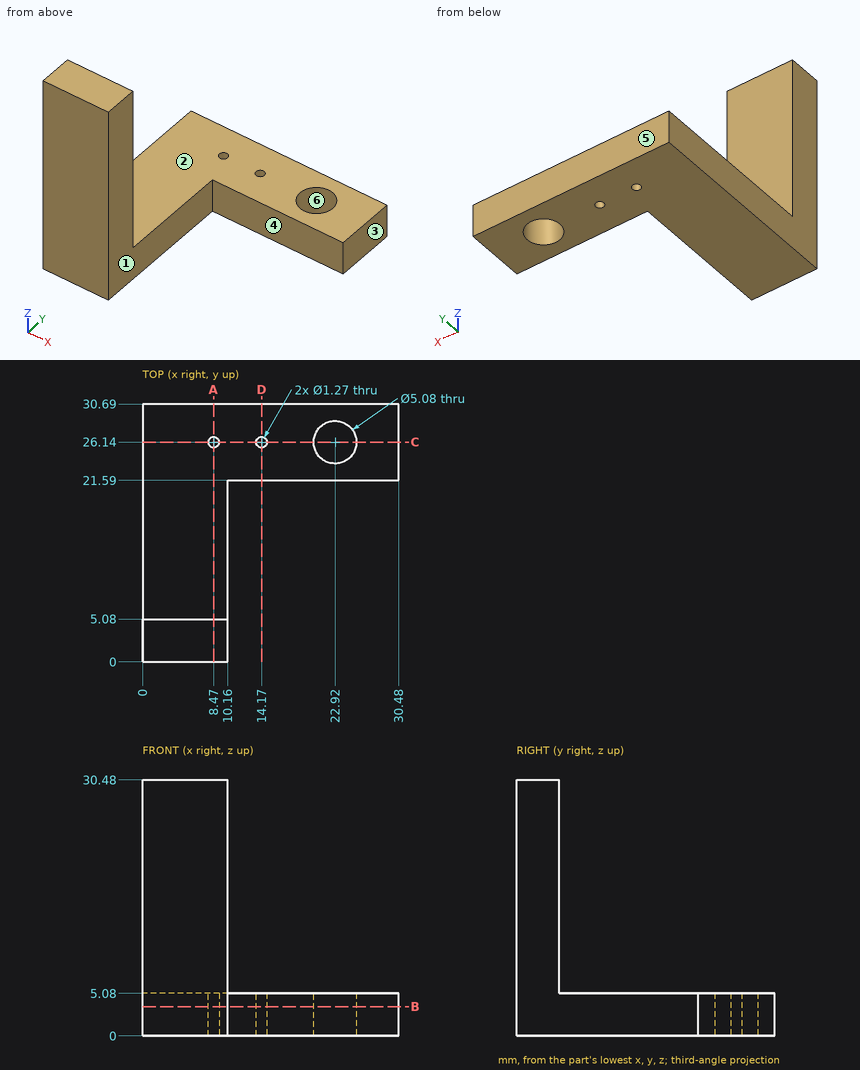
Print and shaded views of the part. All mm, measured from the part's lowest x, y and z. A direction names the side the tool comes from. Give positions to 0.01 mm unless a question says otherwise; leave off trailing zeros. Loops run counter-clockwise (first coordinate to the right, second up) from the corner with the lowest first, then second, coordinate; pieces in that order, holes last. Notation, with made-up numbers: (50.5, 1.5) - (67.5, 1.5) arc R29 cw to (67.5, 38.5) - close; hole circle Ø2 at (-15, -6.75). An arc over 180 degrees is marked (long way). One line per item, written item: value. Start each with the question number.
1. Slice it at D-D (x = 14.17). List the corners of the cut face in (y, z) (3 decimals).
2. Pin check, flat tips, straight feed: pin 1 (3 mm diameter, centred on x = 13, z = 7, fed in from -Y); pin 2 (2 mm diameter, centred on x = 8.47, y = 26.14, fed in from +Z); pin 3 (4 mm diameter, centred on x = 23, z = 3, fed in from -Y); pin 4 (5 mm diameter, centred on x = 3, z = 12, fed in from +Y). Stop position of each tip, or through.
3. Slice it at B-B (z = 3.5). List the corners of the cut face in (x, y) (3 decimals).
4. Probe L1, parallel to Y at x = 22.92, z = 3.4; L2, parallel to Y at x = 8.47, z = 1.8 (3 decimals); L3, parallel to X at y = 26, z = 2. List the from-to ranges inside material, lowest first. Write a range as from..to.
5. Slice it at A-A (x = 8.47). List the corners of the cut face in (y, z) (3 decimals), plus the area to 3 significant figures.
6. Pull direction Y, two halves, no side cores. Call the marked faces 4, 5 and 6: pulls with the +Y half, pulls with the -Y half, needs draft (parallel to the pull), parting line crosses it, or undercut.
7. Which spindle directions (+Z, -Z, +X, -X, +Y, -Y) get a long thin tool onto all of the face, cutting with end or side? Do the marked faces 1, 2 and 3. Say none if no direction does.
8. Slice it at C-C (y = 26.14). List the corners of the cut face in (x, z) (3 decimals), plus the area to 3 significant figures.
Solution:
1. outline: (21.59, 0) - (25.505, 0) - (25.505, 5.08) - (21.59, 5.08) - close; (26.775, 0) - (30.69, 0) - (30.69, 5.08) - (26.775, 5.08) - close
2. pin 1: passes through
2. pin 2: stops at z = 5.08
2. pin 3: stops at y = 21.59
2. pin 4: stops at y = 5.08
3. outline: (0, 0) - (10.16, 0) - (10.16, 21.59) - (30.48, 21.59) - (30.48, 30.69) - (0, 30.69) - close; hole circle Ø1.27 at (8.47, 26.14); hole circle Ø1.27 at (14.17, 26.14); hole circle Ø5.08 at (22.92, 26.14)
4. L1: y = 21.59..23.6, 28.68..30.69
4. L2: y = 0..25.505, 26.775..30.69
4. L3: x = 0..7.85, 9.09..13.55, 14.79..20.38, 25.46..30.48
5. outline: (0, 0) - (25.505, 0) - (25.505, 5.08) - (5.08, 5.08) - (5.08, 30.48) - (0, 30.48) - close; (26.775, 0) - (30.69, 0) - (30.69, 5.08) - (26.775, 5.08) - close
5. area: 278 mm^2
6. face 4: pulls with the -Y half
6. face 5: pulls with the +Y half
6. face 6: undercut
7. face 1: +Z, -Z, +X, -Y
7. face 2: +Z, +X, -X, +Y
7. face 3: +Z, -Z, +X, +Y, -Y
8. outline: (0, 0) - (7.835, 0) - (7.835, 5.08) - (0, 5.08) - close; (9.105, 0) - (13.535, 0) - (13.535, 5.08) - (9.105, 5.08) - close; (14.805, 0) - (20.38, 0) - (20.38, 5.08) - (14.805, 5.08) - close; (25.46, 0) - (30.48, 0) - (30.48, 5.08) - (25.46, 5.08) - close
8. area: 116 mm^2
